from build123d import *

# Parameters (mm, degrees)
SKETCH1_R           = 19.05
BOSS_EXTRUDE1_DEPTH = 69.596
SKETCH2_R           = 3.175
CUT_EXTRUDE1_DEPTH  = 63.5


with BuildPart() as part:
    # Sketch1 → Boss-Extrude1 (new body)
    with BuildSketch(Plane.XY):
        with BuildLine():
            Line((82.55, 0), (-82.55, 0))
            Line((-82.55, 0), (-82.55, -7.9502))
            Line((-82.55, -7.9502), (-39.7002, -7.9502))
            ThreePointArc((-39.7002, -7.9502), (-30.719943879, -11.669943879), (-27.0002, -20.6502))
            Line((-27.0002, -20.6502), (-27.0002, -33.3502))
            ThreePointArc((-27.0002, -33.3502), (-19.092024562, -52.442224464), (-1.39e-07, -60.3504))
            ThreePointArc((-1.39e-07, -60.3504), (19.092024464, -52.442224562), (27.0002, -33.3502))
            Line((27.0002, -33.3502), (27.0002, -20.6502))
            ThreePointArc((27.0002, -20.6502), (30.719943879, -11.669943879), (39.7002, -7.9502))
            Line((39.7002, -7.9502), (82.55, -7.9502))
            Line((82.55, -7.9502), (82.55, 0))
        make_face()
        with Locations((0, -33.3502)):
            Circle(SKETCH1_R, mode=Mode.SUBTRACT)
    extrude(amount=BOSS_EXTRUDE1_DEPTH)

    # Sketch2 → Cut-Extrude1 (cut)
    with BuildSketch(Plane(origin=(0, 0, 0), x_dir=(1, 0, 0), z_dir=(0, 1, 0))):
        with Locations(Location((63.5, -15.875, 0), (0, 0, 180))):
            Circle(SKETCH2_R)
        with Locations(Location((63.5, -47.625, 0), (0, 0, 180))):
            Circle(SKETCH2_R)
        with Locations(Location((-63.5, -47.625, 0), (0, 0, 270))):
            Circle(SKETCH2_R)
        with Locations(Location((-63.5, -15.875, 0), (0, 0, 270))):
            Circle(SKETCH2_R)
    extrude(amount=-CUT_EXTRUDE1_DEPTH, mode=Mode.SUBTRACT)


solid = part.part
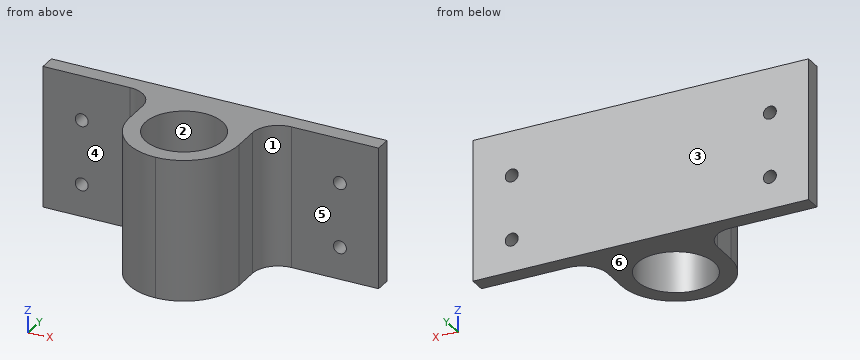
Source: CAD feature listing. Evaluate the final solid. Frame: model axes, mm. Face numbers are marked on the shaded views. A direction names the side the tool comes from. Round coordinates to 2 decimals unless told otherwise and drop trailing zeros. Loops run counter-clockwise (first coordinate to the right, second up) from the corner with the lowest first, then second, coordinate; pieces in that order, holes last. Notation, with made-up numbers: (-31.5, 37.5) - (-7.5, 37.5) arc R33 ccw to (-7.5, 72.5) - close; hole circle Ø4 at (-16.75, 62). An arc over 180 degrees is marked (long way). Write item = value, one per line. Start each with the question number.
Item 1: Section query C-C on x = 11. Output: boundary loops of the cut face in (y, z), plus the area to 3 significant figures.
Item 2: First-contact query: pin 1 Ø2 at (x, z) = (16, 39.5) entering from +Y; pin 2 Ø1 at (x, z) = (12.5, 29) entering from -Y; pin 3 Ø13 at (x, z) = (-57.5, 33.5) entering from -Y; pin 4 Ø12 at (x, z) = (-37, 61) entering from -Y. Flat tips, straight axial feed; report the tip coordinate or a pass-through.
Item 3: Section query A-A on x = -63.5. Output: boundary loops of the cut face in (y, z).
Item 4: Reachability of the marked faces 4, 5 and 6 from +Z, -Z, +X, -X, +Y, -Y: full face, straight path, thin tool, end or side. Return the list, or none.
Item 5: Mould query, pull axis X, two halves, no side actions, for the marked faces 1, 2 and 3. Classes: released by +X, released by -X, zero draft, split by the parting line, or undercut.
Item 6: Section query B-B on z = 42. Output: boundary loops of the cut face in (x, y), plus the area to 3 significant figures.
Item 7: Section query D-D on y = -46. Output: boundary loops of the cut face in (x, z).
Item 8: Material intervals for line 1 (Y direction, x = 0, z = 54); line 2 (X direction, y = -33, z = 9); line 3 (Y direction, x = 47.5, z = 59.5), sorted ascending.
Results list:
q1.outline = (-58.01, 0) - (-48.9, 0) - (-48.9, 69.6) - (-58.01, 69.6) - close; (-17.8, 0) - (0, 0) - (0, 69.6) - (-17.8, 69.6) - close
q1.area = 1,870 mm²
q2.pin_1 = 0
q2.pin_2 = -57.54
q2.pin_3 = -7.95
q2.pin_4 = -11.4
q3.outline = (-7.95, 0) - (0, 0) - (0, 12.7) - (-7.95, 12.7) - close; (-7.95, 19.05) - (0, 19.05) - (0, 44.45) - (-7.95, 44.45) - close; (-7.95, 50.8) - (0, 50.8) - (0, 69.6) - (-7.95, 69.6) - close
q4.face_4 = +Z, -Z, -X, -Y
q4.face_5 = +Z, -Z, +X, -Y
q4.face_6 = -Z, +X, -X, +Y, -Y
q5.face_1 = released by +X
q5.face_2 = undercut
q5.face_3 = zero draft
q6.outline = (-82.55, -7.95) - (-39.7, -7.95) arc R12.7 cw to (-27, -20.65) - (-27, -33.35) arc R27 ccw to (27, -33.35) - (27, -20.65) arc R12.7 cw to (39.7, -7.95) - (82.55, -7.95) - (82.55, 0) - (-82.55, 0) - close; hole circle Ø38.1 at (0, -33.35)
q6.area = 2,760 mm²
q7.outline = (-23.85, 0) - (-14.24, 0) - (-14.24, 69.6) - (-23.85, 69.6) - close; (14.24, 0) - (23.85, 0) - (23.85, 69.6) - (14.24, 69.6) - close
q8.line_1 = -60.35 to -52.4, -14.3 to 0
q8.line_2 = -27 to -19.05, 19.05 to 27
q8.line_3 = -7.95 to 0
